Geometry check sheet. Reference: the model listing, model coordinates, mm. A direction names the side the tool comes from. Give positions to 0.01 mm unless a question says otherwise; leave off trailing zeros. Order: outer loops, then holes, each group sorted by start corner. A loop starts at its lowest first (then second) coordinate and runs counter-clockwise, first axis right, second up.
```python
from build123d import *

# Parameters (mm, degrees)
SKETCH_1_R          = 4.85
EXTRUDE_1_DEPTH     = 1.45
EXTRUDE_2_DEPTH     = 2.95
SKETCH_3_R          = 1.7
CUT_EXTRUDE_1_DEPTH = 39.592535488
FILLET_1_R          = 0.5
FILLET_2_R          = 0.5
FILLET_3_R          = 0.3


with BuildPart() as part:
    # 草图1 → 凸台-拉伸1 (new body)
    with BuildSketch(Plane(origin=(0, 0, 0), x_dir=(1, 0, 0), z_dir=(0, 1, 0))):
        with Locations(Location((33.182897542, 0, 0), (0, 0, 270))):
            Circle(SKETCH_1_R)
    extrude(amount=EXTRUDE_1_DEPTH)

    # 草图2 → 凸台-拉伸2 (add)
    with BuildSketch(Plane(origin=(0, 1.45, 0), x_dir=(1, 0, 0), z_dir=(0, 1, 0))):
        Polygon((37.108879372, 0), (35.145888457, 3.4), (31.219906626, 3.4), (29.256915711, 0), (31.219906626, -3.4), (35.145888457, -3.4), align=None)
    extrude(amount=EXTRUDE_2_DEPTH)

    # 草图3 → 切除-拉伸1 (cut, through all)
    with BuildSketch(Plane(origin=(0, 4.4, 0), x_dir=(1, 0, 0), z_dir=(0, 1, 0))):
        with Locations(Location((33.182897542, 0, 0), (0, 0, 270))):
            Circle(SKETCH_3_R)
    extrude(amount=-CUT_EXTRUDE_1_DEPTH, mode=Mode.SUBTRACT)

    # 圆角1
    fillet_1_edges = [part.edges().sort_by_distance(p)[0] for p in [
        (36.127383914, 4.4, 1.7),
        (36.127383914, 4.4, -1.7),
        (33.182897542, 4.4, -3.4),
        (30.238411169, 4.4, -1.7),
        (30.238411169, 4.4, 1.7),
        (33.182897542, 4.4, 3.4),
    ]]
    fillet(fillet_1_edges, radius=FILLET_1_R)

    # 圆角2
    fillet_2_edges = [part.edges().sort_by_distance(p)[0] for p in [
        (33.182897542, 1.45, -4.85),
    ]]
    fillet(fillet_2_edges, radius=FILLET_2_R)

    # 圆角3
    fillet_3_edges = [part.edges().sort_by_distance(p)[0] for p in [
        (36.127383914, 1.45, 1.7),
        (36.127383914, 1.45, -1.7),
        (33.182897542, 1.45, -3.4),
        (30.238411169, 1.45, -1.7),
        (30.238411169, 1.45, 1.7),
        (33.182897542, 1.45, 3.4),
    ]]
    fillet(fillet_3_edges, radius=FILLET_3_R)


solid = part.part
```
Q1. Cross-section at A-A, the plane y = 2.3. Record the boundary of the cut face in (x, z), and give its area (3 significant figures).
Q2. Cross-section at B-B, the plane y = 0.5. Record the boundary of the cut face in (x, z), and give its area (3 significant figures).
Q3. Access from +Z, -Z, +X, -X, +Y, -Y to the whole of each face (thin tool, end or side, straight path). Record for faces 4 (the face through (30.225, 2.81, 1.676)), 5 (the face through (33, 3, -3.4)), 6 (the face through (36.114, 2.81, 1.724)), 7 (the face through (30.25, 2.81, -1.72)).
Q4. Gauge pin test, flat ends, axial feed: P1, Ø5, axis at x = 33.5, z = -0.5, coming from the -Y side; P2, Ø2, axis at x = 30.5, y = 2, coming from the +Z side; P3, Ø1.7, axis at x = 33, y = 3, coming from the +Z side; P4, Ø1.7, axis at x = 33.5, y = 3.5, coming from the -Z side. Record the tip position at first contact, or that the pin passes through.
Q5. Thickness scan on L1, parallel to Y at x = 30.5, z = 1.25; L2, parallel to Y at x = 35.5, z = -3.75; L3, parallel to Z at x = 32.75, y = 3.15. Record the ranges inside material, lowest first.
Q6. Release check for a two-part mould opening along Z. For faces 1 (the face through (31.523, 2.231, -0.369)), 2 (the face through (30.376, 4.25, 1.653)), 3 (the face through (35, 4.4, -1)) record: pulls with the +Z half, pulls with the -Z half, needs draft (parallel to the pull), parting line crosses it, or undercut.
Answers follow:
1. outline: (29.26, 0) - (31.22, -3.4) - (35.15, -3.4) - (37.11, 0) - (35.15, 3.4) - (31.22, 3.4) - close; hole circle Ø3.4 at (33.18, 0)
1. area: 31.0 mm2
2. outline: circle Ø9.7 at (33.18, 0); hole circle Ø3.4 at (33.18, 0)
2. area: 64.8 mm2
3. face 4: +Z, -X, +Y
3. face 5: -Z, +X, -X, +Y
3. face 6: +Z, +X, +Y
3. face 7: -Z, -X, +Y
4. P1: stops at y = 0
4. P2: stops at z = 4.31
4. P3: stops at z = 3.4
4. P4: stops at z = -3.4
5. L1: y = 0 to 4.4
5. L2: y = 0 to 1.45
5. L3: z = -3.4 to -1.64, 1.64 to 3.4
6. face 1: undercut
6. face 2: pulls with the +Z half
6. face 3: needs draft
